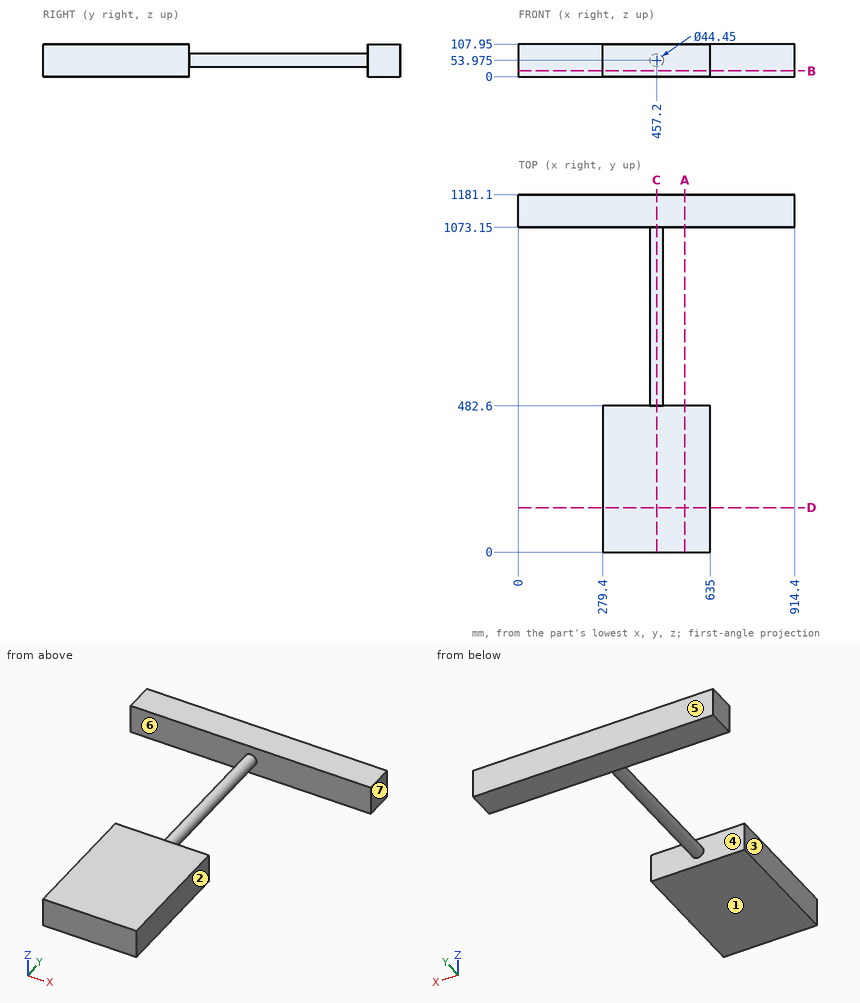
Study the drawing (mm; zero at the part's minimum x, y, z) and answer. A direction names the side the tool comes from. Coordinates: 2 decimals unless noted, no trailing zeros. Order: outer loops, then holes, each group sorted by start corner. A loop starts at its lowest first (then second) coordinate and runs counter-clockwise, first axis right, second up. Notation, with made-up numbers: M 66,-22 L 94,-22 A19 cw 94,3 Z; hole C 1,-0.5 d10. An arc over 180 degrees is marked long. Answer as a JSON object with one key per item and string values. Group by question number.
1. Determine the mould class of the marked faces 4, 5, 6 and 7 for opening direction Y: released by +Y, released by -Y, zero draft, split by the parting line, or undercut.
2. Straight lines are drawn through the part: line 1 (Y direction, x = 535, z = 68); line 2 (Y direction, x = 752, z = 65.5); line 3 (Z direction, x = 455.5, y = 764). For each, find the intervals that lie inside material, in ascending order.
3. Section D-D on y = 147 is taken. Write down the section's boundary in (x, z).
4. Flat-ended cylindrical pins translate along their axes: P1, Ø4, axis at y = 787, z = 67.5, coming from the +X side; P2, Ø2, axis at y = 988, z = 57, coming from the -X side. Find the tip coordinate at first contact, or state that the pin passes through.
5. Section B-B on z = 19 is taken. Write down the section's boundary in (x, y).
6. A tool of negligible diameter and unlimited length cuts with its end or side. For the marked faces 1, 2 and 3, from which of +Z, -Z, +X, -X, +Y, -Y can it reach the whole face along a straight path? Write none if from no direction.
7. Section A-A on x = 550 is taken. Write down the section's boundary in (y, z), then the cut area to 4 significant figures.
8. Section C-C on x = 457.2 is taken. Write down the section's boundary in (y, z), then the cut area to 3 significant figures.
Values follow:
{
 "1": {"face 4": "undercut", "face 5": "released by +Y", "face 6": "undercut", "face 7": "zero draft"},
 "2": {"line 1": "0 to 482.6, 1073.15 to 1181.1", "line 2": "1073.15 to 1181.1", "line 3": "31.82 to 76.13"},
 "3": {"outline": "M 279.4,0 L 635,0 L 635,107.95 L 279.4,107.95 Z"},
 "4": {"P1": "x = 476.2", "P2": "x = 435.07"},
 "5": {"outline": "M 0,1073.15 L 914.4,1073.15 L 914.4,1181.1 L 0,1181.1 Z; M 279.4,0 L 635,0 L 635,482.6 L 279.4,482.6 Z"},
 "6": {"face 1": "-Z, +X, -X, +Y, -Y", "face 2": "+Z, -Z, +X, -Y", "face 3": "+Z, -Z, -X, -Y"},
 "7": {"outline": "M 0,0 L 482.6,0 L 482.6,107.95 L 0,107.95 Z; M 1073.15,0 L 1181.1,0 L 1181.1,107.95 L 1073.15,107.95 Z", "area": "63,750 mm2"},
 "8": {"outline": "M 0,0 L 482.6,0 L 482.6,31.75 L 1073.15,31.75 L 1073.15,0 L 1181.1,0 L 1181.1,107.95 L 1073.15,107.95 L 1073.15,76.2 L 482.6,76.2 L 482.6,107.95 L 0,107.95 Z", "area": "90,000 mm2"}
}
